The drawing under review shows one solid part. Ordinate dimensions are in mm from its lowest x, y, z. Coordinates: 2 decimals unless noted, no trailing zeros. Write each loop counter-clockwise with the first axis right and the second up, starting at its lowest first coordinate (ties: lowest second). Pieces come first, ordered by that corner, then holes. Notation, with made-up numbers: (29.5, 86) - (40.5, 86) arc R18 cw to (40.5, 119) - close; hole circle Ø3 at (81, 65.5). An arc over 180 degrees is marked (long way). Use a Markdown table: item, result.
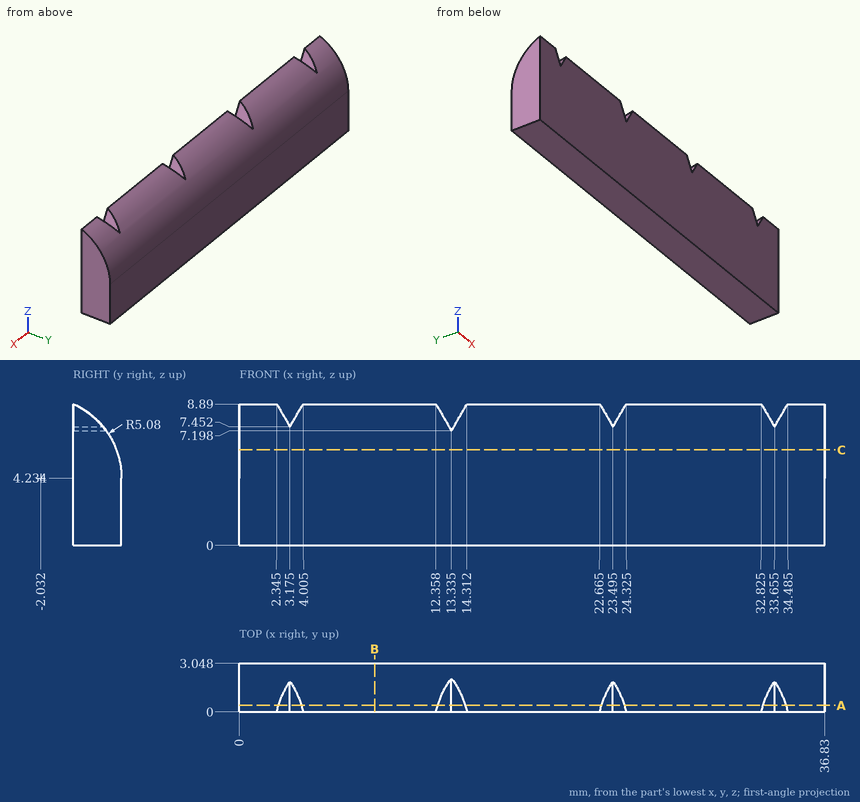
(1) Take a section at A-A on y = 0.4. Write out the cut boundary in (x, z) (1 decimal).
Determined:
| item | result |
|---|---|
| outline | (0, 0) - (36.8, 0) - (36.8, 8.7) - (34.4, 8.7) - (33.7, 7.5) - (32.9, 8.7) - (24.2, 8.7) - (23.5, 7.5) - (22.8, 8.7) - (14.2, 8.7) - (13.3, 7.2) - (12.5, 8.7) - (3.9, 8.7) - (3.2, 7.5) - (2.5, 8.7) - (0, 8.7) - close |
(2) Take a section at B-B on x = 8.5. Write out the cut boundary in (y, z).
Determined:
| item | result |
|---|---|
| outline | (0, 0) - (3.05, 0) - (3.05, 4.23) arc R5.08 ccw to (0, 8.89) - close |
(3) For pin 1 (1 mm diameter, centred on x = 16.5, y = 2.5, fed in from -Z), flat-tipped, find the tip position at first contact; note if it passes through.
Determined:
| item | result |
|---|---|
| pin 1 | z = 0 |
(4) Take a section at C-C on z = 6. Write out the cut boundary in (x, y), and give its area (3 significant figures).
Determined:
| item | result |
|---|---|
| outline | (0, 0) - (36.83, 0) - (36.83, 2.73) - (0, 2.73) - close |
| area | 101 mm2 |
(5) For L1, parallel to Z at x = 35, y = 1.9; L2, parallel to Y at x = 28, z = 8.25; L3, parallel to Z at x = 8.5, y = 1.25, list the stretches that pass through material, from the lowest coordinate up. Write a range as from..to.
Determined:
| item | result |
|---|---|
| L1 | 0..7.45 |
| L2 | 0..1.08 |
| L3 | 0..8.11 |
